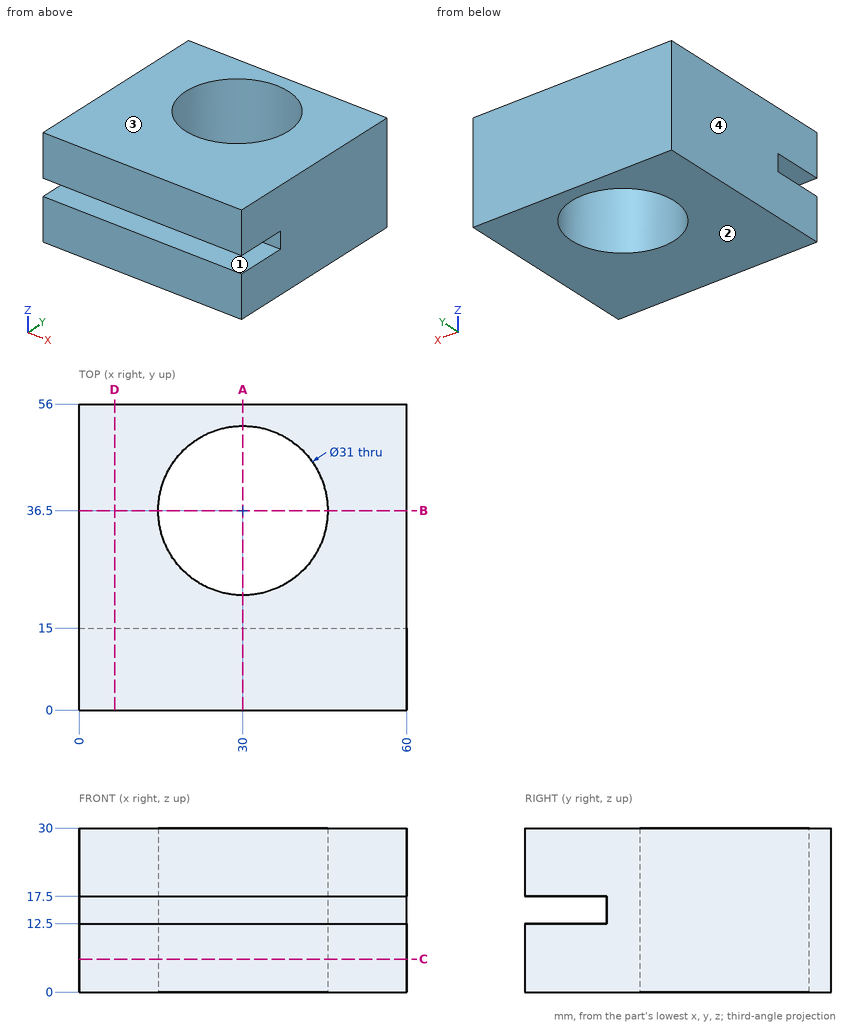
Check sheet for the drawn part. Datum: minimum x, y, z corner. Units: mm. Coordinates: 2 decimals unless noted, no trailing zeros. Order: outer loops, then holes, each group sorted by start corner. A loop starts at its lowest first (then second) coordinate and runs counter-clockwise, first axis right, second up. Notation, with made-up numbers: M 11,22 L 43,22 A31 cw 43,60 Z; hole C -5,85 d8. An arc over 180 degrees is marked long. One line per question, with ' | ' between items. Start each with the question number.
Item 1: Cross-section at C-C on z = 6. Enter the section's corners in (x, y), then the cut area to 3 significant figures.
Item 2: Gauge pin test, flat end, axial feed: pin 1 (2.5 mm diameter, centred on x = 28, z = 15, fed in from -Y). Record the tip position at first contact, or that the pin passes through.
Item 3: Cross-section at B-B on y = 36.5. Enter the section's corners in (x, z), then the cut area to 3 significant figures.
Item 4: Cross-section at D-D on x = 6.5. Enter the section's corners in (y, z), then the cut area to 4 significant figures.
Item 5: Cross-section at A-A on x = 30. Enter the section's corners in (y, z), then the cut area to 3 significant figures.
Item 6: Material ranges on L1, parallel to Z at x = 11, y = 11.5; L2, parallel to X at y = 36.5, z = 23.5; L3, parallel to Y at x = 17.5, z = 19, recorded low to high. Write a range as [from, to].
Item 7: Draft check along Z on the marked faces 1, 2, 3 and 4. Enter one of: pulls with the +Z half, pulls with the -Z half, needs draft (parallel to the pull), parting line crosses it, or undercut.
Findings:
1) outline: M 0,0 L 60,0 L 60,56 L 0,56 Z; hole C 30,36.5 d31 | area: 2,610 mm²
2) pin 1: stops at y = 15
3) outline: M 0,0 L 14.5,0 L 14.5,30 L 0,30 Z; M 45.5,0 L 60,0 L 60,30 L 45.5,30 Z | area: 870 mm²
4) outline: M 0,0 L 56,0 L 56,30 L 0,30 L 0,17.5 L 15,17.5 L 15,12.5 L 0,12.5 Z | area: 1,605 mm²
5) outline: M 0,0 L 21,0 L 21,30 L 0,30 L 0,17.5 L 15,17.5 L 15,12.5 L 0,12.5 Z; M 52,0 L 56,0 L 56,30 L 52,30 Z | area: 675 mm²
6) L1: z = [0, 12.5], [17.5, 30] | L2: x = [0, 14.5], [45.5, 60] | L3: y = [0, 27.33], [45.67, 56]
7) face 1: undercut | face 2: pulls with the -Z half | face 3: pulls with the +Z half | face 4: needs draft
